from build123d import *

# Parameters (mm, degrees)
BOSS_EXTRUDE1_DEPTH = 0.45
SKETCH2_W           = 11
SKETCH2_H           = 0.5
BOSS_EXTRUDE2_DEPTH = 0.25
BOSS_EXTRUDE3_DEPTH = 8
BOSS_EXTRUDE4_DEPTH = 0.25
SKETCH5_W           = 11
SKETCH5_H           = 0.8
BOSS_EXTRUDE5_DEPTH = 4


with BuildPart() as part:
    # Sketch1 → Boss-Extrude1 (new body)
    with BuildSketch(Plane.XY):
        Polygon((19.629909152, 0), (9.814954576, 17), (-9.814954576, 17), (-19.629909152, 0), (-9.814954576, -17), (9.814954576, -17), align=None)
    extrude(amount=BOSS_EXTRUDE1_DEPTH)

    # Sketch2 → Boss-Extrude2 (add)
    with BuildSketch(Plane.XY):
        with Locations((0, 17.25)):
            Rectangle(SKETCH2_W, SKETCH2_H)
        Polygon((12.405444566, 13.513139721), (17.905444566, 3.986860279), (17.472431864, 3.736860279), (11.972431864, 13.263139721), align=None)
        Polygon((17.905444566, -3.986860279), (12.405444566, -13.513139721), (11.972431864, -13.263139721), (17.472431864, -3.736860279), align=None)
        with Locations((0, -17.25)):
            Rectangle(SKETCH2_W, SKETCH2_H)
        Polygon((-12.405444566, -13.513139721), (-17.905444566, -3.986860279), (-17.472431864, -3.736860279), (-11.972431864, -13.263139721), align=None)
        Polygon((-17.905444566, 3.986860279), (-12.405444566, 13.513139721), (-11.972431864, 13.263139721), (-17.472431864, 3.736860279), align=None)
    extrude(amount=BOSS_EXTRUDE2_DEPTH)

    # Sketch3 → Boss-Extrude3 (add)
    with BuildSketch(Plane.XY):
        Polygon((-11.972431864, 13.263139721), (-10.240381057, 12.263139721), (-8.660254038, 15), (-5.5, 15), (-5.5, 17), (-7.5, 17), (-9.814954576, 17), (-10.972431864, 14.995190528), align=None)
        Polygon((5.5, 17), (5.5, 15), (8.660254038, 15), (10.240381057, 12.263139721), (11.972431864, 13.263139721), (10.972431864, 14.995190528), (9.814954576, 17), (7.5, 17), align=None)
        Polygon((17.472431864, 3.736860279), (15.740381057, 2.736860279), (17.320508076, 0), (15.740381057, -2.736860279), (17.472431864, -3.736860279), (18.472431864, -2.004809472), (19.629909152, 0), (18.472431864, 2.004809472), align=None)
        Polygon((11.972431864, -13.263139721), (10.240381057, -12.263139721), (8.660254038, -15), (5.5, -15), (5.5, -17), (7.5, -17), (9.814954576, -17), (10.972431864, -14.995190528), align=None)
        Polygon((-5.5, -17), (-5.5, -15), (-8.660254038, -15), (-10.240381057, -12.263139721), (-11.972431864, -13.263139721), (-10.972431864, -14.995190528), (-9.814954576, -17), (-7.5, -17), align=None)
        Polygon((-17.472431864, -3.736860279), (-15.740381057, -2.736860279), (-17.320508076, 0), (-15.740381057, 2.736860279), (-17.472431864, 3.736860279), (-18.472431864, 2.004809472), (-19.629909152, 0), (-18.472431864, -2.004809472), align=None)
    extrude(amount=BOSS_EXTRUDE3_DEPTH)

    # Sketch4 → Boss-Extrude4 (add)
    with BuildSketch(Plane.XY):
        Polygon((21.939310229, 0), (10.969655115, 19), (-10.969655115, 19), (-21.939310229, 0), (-10.969655115, -19), (10.969655115, -19), align=None)
    extrude(amount=BOSS_EXTRUDE4_DEPTH)

    # Sketch5 → Boss-Extrude5 (add)
    with BuildSketch(Plane.XY.offset(0.45)):
        with Locations((0, 16.6)):
            Rectangle(SKETCH5_W, SKETCH5_H)
        Polygon((11.972431864, 13.263139721), (17.472431864, 3.736860279), (16.779611541, 3.336860279), (11.279611541, 12.863139721), align=None)
        Polygon((17.472431864, -3.736860279), (11.972431864, -13.263139721), (11.279611541, -12.863139721), (16.779611541, -3.336860279), align=None)
        with Locations((0, -16.6)):
            Rectangle(SKETCH5_W, SKETCH5_H)
        Polygon((-11.972431864, -13.263139721), (-17.472431864, -3.736860279), (-16.779611541, -3.336860279), (-11.279611541, -12.863139721), align=None)
        Polygon((-17.472431864, 3.736860279), (-11.972431864, 13.263139721), (-11.279611541, 12.863139721), (-16.779611541, 3.336860279), align=None)
    extrude(amount=BOSS_EXTRUDE5_DEPTH)


solid = part.part
Source: CAD feature listing. Evaluate the final solid. Frame: model axes, mm. A direction names the side the tool comes from. Round coordinates to 2 decimals unless told otherwise and drop trailing zeros. Order: outer loops, then holes, each group sorted by start corner. A loop starts at its lowest first (then second) coordinate and runs counter-clockwise, first axis right, second up. Notation, with made-up numbers: (85, 18.25) - (141, 18.25) arc R16 ccw to (141, 25.25) - close; hole circle Ø5 at (36.25, -30.5). An arc over 180 degrees is marked (long way). Use a Markdown table: item, result. Add a question column.
1. Section query B-B (y = 15.5). Return the cut outline in (x, z).
2. Section query A-A (x = -2). Return the cut outline in (y, z).
3. First-contact query: pin 1 (0.9 mm diameter, centred on x = 7.5, z = 5.5, fed in from +Y); pin 2 (3 mm diameter, centred on x = -2, z = 2.5, fed in from -Y); pin 3 (0.6 mm diameter, centred on y = 16.5, z = 6, fed in from -X). Flat tips, straight axial feed; report the tip coordinate or a pass-through.
4. Set-up query: faces 1 (the flat face through (-9, -15, 8)), 2 (the flat face through (16.4, -3.12, 5.01)). Return all of +Z, -Z, +X, -X, +Y, -Y with unobstructed straight access to the full face (end or side cutting, diameter ignored); none if empty.
5. Section query D-D (x = 6.5). Return the cut outline in (y, z), then the cut area to 3 significant figures.
6. Section query C-C (z = 6). Give the number of separate pieces and of enclosed holes in the cut face, then the cut area to 3 significant figures.
7. Line query: probe 1 along Y at (x, z) = (0.5, 3); probe 2 along Y at (x, z) = (6.5, 7); probe 3 along Z at (x, y) = (-0.5, 12). Output: solid intervals per line, ascending.
8. Mould query, pull axis X, two halves, no side actions, for faces 3 (the flat face through (0, -17, 3)), 4 (the flat face through (-16.426, -3.133, 5.011)). Classes: +X half, -X half, draft (parallel to the pull), parting line (faces both ways), or undercut.
Derived:
| question | item | result |
|---|---|---|
| 1 | outline | (-12.99, 0) - (12.99, 0) - (12.99, 0.25) - (10.68, 0.25) - (10.68, 8) - (5.5, 8) - (5.5, 0.45) - (-5.5, 0.45) - (-5.5, 8) - (-10.68, 8) - (-10.68, 0.25) - (-12.99, 0.25) - close |
| 2 | outline | (-19, 0) - (19, 0) - (19, 0.25) - (17, 0.25) - (17, 4.45) - (16.2, 4.45) - (16.2, 0.45) - (-16.2, 0.45) - (-16.2, 4.45) - (-17, 4.45) - (-17, 0.25) - (-19, 0.25) - close |
| 3 | pin 1 | y = 17 |
| 3 | pin 2 | y = -17 |
| 3 | pin 3 | x = -10.28 |
| 4 | face 1 | +Z, +X, -X, +Y, -Y |
| 4 | face 2 | +Z |
| 5 | outline | (-19, 0) - (19, 0) - (19, 0.25) - (17, 0.25) - (17, 8) - (15, 8) - (15, 0.45) - (-15, 0.45) - (-15, 8) - (-17, 8) - (-17, 0.25) - (-19, 0.25) - close |
| 5 | area | 46.5 mm2 |
| 6 | separate pieces | 6 |
| 6 | enclosed holes | 0 |
| 6 | area | 89.7 mm2 |
| 7 | probe 1 | -17 to -16.2, 16.2 to 17 |
| 7 | probe 2 | -17 to -15, 15 to 17 |
| 7 | probe 3 | 0 to 0.45 |
| 8 | face 3 | draft |
| 8 | face 4 | undercut |
